from build123d import *

# Parameters (mm, degrees)
CHAMFER1_SIZE = 1


with BuildPart() as part:
    # Sketch1 → Revolve1 (revolve)
    with BuildSketch(Plane(origin=(0, 0, 0), x_dir=(0, 0, -1), z_dir=(1, 0, 0)), mode=Mode.PRIVATE) as revolve1_sk:
        Polygon((0, 0), (-13.5, 0), (-13.5, 21.2), (-12.5, 22.2), (-10.5, 22.2), (-10.5, 22.5), (-1, 22.5), (0, 21.5), align=None)
    revolve(revolve1_sk.sketch.rotate(Axis((0, 0, 0), (0, 0, 1)), 90), axis=Axis((0, 0, 0), (0, 0, 1)))

    # Sketch2 → Cut-Revolve1 (revolve, cut)
    with BuildSketch(Plane(origin=(0, 0, 0), x_dir=(0, 0, -1), z_dir=(1, 0, 0)), mode=Mode.PRIVATE) as cut_revolve1_sk:
        Polygon((0, 0), (-13.5, 0), (-13.5, 14), (-10.5, 14), (-10, 14.5), (-9.5, 14), (-7.2, 14), (-6.2, 15), (-6.2, 18), (0, 18), align=None)
    revolve(cut_revolve1_sk.sketch.rotate(Axis((0, 0, 0), (0, 0, 1)), 90), axis=Axis((0, 0, 0), (0, 0, 1)), mode=Mode.SUBTRACT)

    # Chamfer1
    chamfer1_edges = [part.edges().sort_by_distance(p)[0] for p in [
        (18, 0, 0),
        (14, 0, 13.5),
    ]]
    chamfer(chamfer1_edges, length=CHAMFER1_SIZE)


solid = part.part
Source: CAD feature listing. Evaluate the final solid. Frame: model axes, mm. A direction names the side the tool comes from. Coordinates: 2 decimals unless noted, no trailing zeros. Write each loop counter-clockwise with the first axis right and the second up, starting at its lowest first coordinate (ties: lowest second). Pieces come first, ordered by that corner, then holes. Notation, with made-up numbers: M -31,-15.75 L -7,-15.75 A12 ccw -7,4.25 Z; hole C 67,50.25 d3. An arc over 180 degrees is marked long. Use a Markdown table: item, result.
1) Ray query, L1, parallel to Y at x = 0, z = 11.1; L2, parallel to Y at x = 0, z = 8.1; L3, parallel to Z at x = 15, y = 2.5. Return the intervals inside material, ascending.
Conclusion:
| item | result |
|---|---|
| L1 | y = -22.2 to -14, 14 to 22.2 |
| L2 | y = -22.5 to -14, 14 to 22.5 |
| L3 | z = 6.2 to 13.5 |
2) Section C-C, the plane z = 4. Output: boundary loops of the cut face in (x, y).
Conclusion:
| item | result |
|---|---|
| outline | C 0,0 d45; hole C 0,0 d36 |
3) First-contact query: pin 1 Ø2 at (y, z) = (11, 3) entering from -X; pin 2 Ø1 at (x, z) = (-6, 3.5) entering from -Y; pin 3 Ø1.5 at (y, z) = (6.5, 11.5) entering from +X; pin 4 Ø22.5 at (x, y) = (0, 0) entering from +Z. Flat tips, straight axial feed; report the tip coordinate or a pass-through.
Conclusion:
| item | result |
|---|---|
| pin 1 | stops at x = -20.16 |
| pin 2 | stops at y = -21.82 |
| pin 3 | stops at x = 21.44 |
| pin 4 | passes through |
4) Reachability of faces 1 (the flat face through (-5, -14.4, 13.5)), 2 (the flat face through (-4, -15, 6.2)), 3 (the cylindrical face through (2.89, -22.01, 11.49)) from +Z, -Z, +X, -X, +Y, -Y: full face, straight path, thin tool, end or side. Return the list, or none.
Conclusion:
| item | result |
|---|---|
| face 1 | +Z, +X, -X, +Y, -Y |
| face 2 | -Z |
| face 3 | +Z |
5) Mould query, pull axis Y, two halves, no side actions, for faces 4 (the flat face through (-11, 16, 0)), 5 (the cylindrical face through (-6.5, 12.4, 8.3)), 6 (the cylindrical face through (-10.382, 19.961, 5.684)). Classes: pulls with the +Y half, pulls with the -Y half, needs draft (parallel to the pull), parting line crosses it, or undercut.
Conclusion:
| item | result |
|---|---|
| face 4 | needs draft |
| face 5 | undercut |
| face 6 | parting line crosses it |
